Here's how the part is built. I have some questions about the finished solid (model axes, mm). Give positions to 0.01 mm unless a question says otherwise; leave off trailing zeros. Loops run counter-clockwise (first coordinate to the right, second up) from the corner with the lowest first, then second, coordinate; pieces in that order, holes last.
Q1. Suppose I cut it at A-A (z = -15). List the corners of the cut face in (x, y) for me.
Q2. I need wall thicknesses on probe 1 along X at (y, z) = (2.35, -15); probe 2 along X at (y, z) = (5.6, -10); probe 3 along Z at (x, y) = (-279, 5.15). Which ranges of each line are inside material? Lowest first, please.
Q3. Suppose I cut it at B-B (x = -183.5). List the corners of the cut face in (y, z) for me, and give its area (3 significant figures).
Q4. Suppose I cut it at C-C (z = -45.5). List the corners of the cut face in (x, y) for me.
Q5. I'm going to push flat-ended pins straight in: P1, Ø6, axis at x = -194, z = -12, coming from the -Y side; P2, Ø1.8, axis at y = 3.5, z = 2.5, coming from the -X side; P3, Ø1.8, axis at y = 2, z = 2.5, coming from the +X side; P4, Ø1.5, axis at y = 5, z = -43, coming from the -X side. Where does each tip first touch, or does it pass through?
Q6. Suppose I cut it at D-D (y = 1.35). Count the separate pieces of the cut face and the enclosed holes in it, and give its area (3 significant figures).
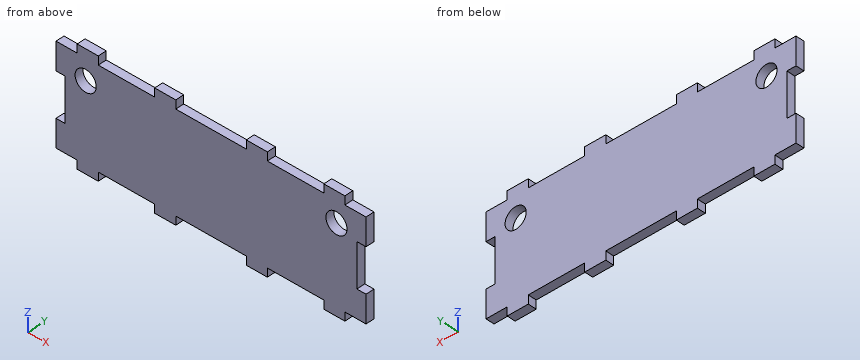
```python
from build123d import *

# Parameters (mm, degrees)
BOSS_EXTRUDE1_DEPTH = 6
CAVITY1_START       = -365.386748432
CAVITY1_OUTLINE_W   = 6
CAVITY1_OUTLINE_H   = 30
CAVITY1_DEPTH       = 6
CAVITY1_START_2     = -151.386748432
CAVITY1_2_OUTLINE_W = 6
CAVITY1_2_OUTLINE_H = 30
CAVITY1_2_DEPTH     = 6
SKETCH2_R           = 7.5
CUT_EXTRUDE1_DEPTH  = 10
SKETCH3_W           = 6.5
SKETCH3_H           = 31
CUT_EXTRUDE2_DEPTH  = 10


# Read off the part's stored shape, not the designer's step: Cavity1
with BuildPart() as part:
    # Sketch1 → Boss-Extrude1 (new body)
    with BuildSketch(Plane(origin=(0, 0, 0), x_dir=(1, 0, 0), z_dir=(0, 1, 0))):
        Polygon((-160.386748432, 70), (-145.386748432, 70), (-145.386748432, 0), (-160.386748432, 0), (-160.386748432, -6), (-175.386748432, -6), (-175.386748432, 0), (-215.386748432, 0), (-215.386748432, -6), (-230.386748432, -6), (-230.386748432, 0), (-280.386748432, 0), (-280.386748432, -6), (-295.386748432, -6), (-295.386748432, 0), (-335.386748432, 0), (-335.386748432, -6), (-350.386748432, -6), (-350.386748432, 0), (-365.386748432, 0), (-365.386748432, 70), (-350.386748432, 70), (-350.386748432, 76), (-335.386748432, 76), (-335.386748432, 70), (-295.386748432, 70), (-295.386748432, 76), (-280.386748432, 76), (-280.386748432, 70), (-230.386748432, 70), (-230.386748432, 76), (-215.386748432, 76), (-215.386748432, 70), (-175.386748432, 70), (-175.386748432, 76), (-160.386748432, 76), align=None)
    extrude(amount=BOSS_EXTRUDE1_DEPTH)

    # Cavity1 outline → Cavity1 (cut)
    with BuildSketch(Plane.YZ.offset(CAVITY1_START)):
        with Locations((3, -35)):
            Rectangle(CAVITY1_OUTLINE_W, CAVITY1_OUTLINE_H)
    extrude(amount=CAVITY1_DEPTH, mode=Mode.SUBTRACT)

    # Cavity1 2 outline → Cavity1 2 (cut)
    with BuildSketch(Plane.YZ.offset(CAVITY1_START_2)):
        with Locations((3, -35)):
            Rectangle(CAVITY1_2_OUTLINE_W, CAVITY1_2_OUTLINE_H)
    extrude(amount=CAVITY1_2_DEPTH, mode=Mode.SUBTRACT)

    # Sketch2 → Cut-Extrude1 (cut)
    with BuildSketch(Plane.XZ):
        with Locations(Location((-166.386748432, -15, 0), (0, 0, 270))):
            Circle(SKETCH2_R)
        with Locations(Location((-344.386748432, -15, 0), (0, 0, 270))):
            Circle(SKETCH2_R)
    extrude(amount=-CUT_EXTRUDE1_DEPTH, mode=Mode.SUBTRACT)

    # Sketch3 → Cut-Extrude2 (cut)
    with BuildSketch(Plane(origin=(0, 6, 0), x_dir=(1, 0, 0), z_dir=(0, 1, 0))):
        with Locations((-148.636748432, 35)):
            Rectangle(SKETCH3_W, SKETCH3_H)
        with Locations((-362.136748432, 35)):
            Rectangle(SKETCH3_W, SKETCH3_H)
    extrude(amount=-CUT_EXTRUDE2_DEPTH, mode=Mode.SUBTRACT)


solid = part.part
```
Solutions:
1. outline: (-365.39, 0) - (-351.89, 0) - (-351.89, 6) - (-365.39, 6) - close; (-336.89, 0) - (-173.89, 0) - (-173.89, 6) - (-336.89, 6) - close; (-158.89, 0) - (-145.39, 0) - (-145.39, 6) - (-158.89, 6) - close
2. probe 1: x = -365.39 to -351.89, -336.89 to -173.89, -158.89 to -145.39
2. probe 2: x = -365.39 to -349.98, -338.8 to -171.98, -160.8 to -145.39
2. probe 3: z = -70 to 0
3. outline: (0, -70) - (6, -70) - (6, 0) - (0, 0) - close
3. area: 420 mm2
4. outline: (-358.89, 0) - (-151.89, 0) - (-151.89, 6) - (-358.89, 6) - close
5. P1: stops at y = 0
5. P2: stops at x = -350.39
5. P3: stops at x = -160.39
5. P4: stops at x = -358.89
6. separate pieces: 1
6. enclosed holes: 2
6. area: 15,400 mm2
